```python
from build123d import *

# Parameters (mm, degrees)
SKETCH_1_W          = 40.5
SKETCH_1_H          = 20.25
EXTRUDE_1_DEPTH     = 9
CUT_EXTRUDE_START   = -1
SKETCH_2_R          = 9.25
CUT_EXTRUDE_1_DEPTH = 9
SKETCH_3_W          = 6.125
SKETCH_3_H          = 8
SKETCH_3_W_2        = 8
SKETCH_3_W_3        = 12.25
SKETCH_3_H_2        = 6.125
CUT_EXTRUDE_2_DEPTH = 1
CHAMFER_1_SIZE      = 1
SKETCH_4_R          = 1.1
SKETCH_4_R_2        = 0.7
SKETCH_4_R_3        = 0.9
SKETCH_4_R_4        = 0.5
CUT_EXTRUDE_3_DEPTH = 7.2
EXTRUDE_2_DEPTH     = 7.8
CUT_EXTRUDE_4_DEPTH = 7.8
FILLET_1_R          = 0.3


with BuildPart() as part:
    # Эскиз1 → Бобышка-Вытянуть1 (new body)
    with BuildSketch(Plane.XY):
        Rectangle(SKETCH_1_W, SKETCH_1_H)
    extrude(amount=EXTRUDE_1_DEPTH)

    # Эскиз2 → Вырез-Вытянуть1 (cut)
    with BuildSketch(Plane.XY.offset(9).offset(CUT_EXTRUDE_START)):
        with Locations((-10.125, 0)):
            Circle(SKETCH_2_R)
        with Locations((10.125, 0)):
            Circle(SKETCH_2_R)
    extrude(amount=-CUT_EXTRUDE_1_DEPTH, mode=Mode.SUBTRACT)

    # Эскиз3 → Вырез-Вытянуть2 (cut)
    with BuildSketch(Plane.XY.offset(9)):
        with Locations((-17.1875, 0)):
            Rectangle(SKETCH_3_W, SKETCH_3_H)
        with Locations((-10.125, 0)):
            Rectangle(SKETCH_3_W_2, SKETCH_3_H)
        Rectangle(SKETCH_3_W_3, SKETCH_3_H)
        with Locations((10.125, 0)):
            Rectangle(SKETCH_3_W_2, SKETCH_3_H)
        with Locations((17.1875, 0)):
            Rectangle(SKETCH_3_W, SKETCH_3_H)
        with Locations((10.125, 7.0625)):
            Rectangle(SKETCH_3_W_2, SKETCH_3_H_2)
        with Locations((-10.125, 7.0625)):
            Rectangle(SKETCH_3_W_2, SKETCH_3_H_2)
        with Locations((-10.125, -7.0625)):
            Rectangle(SKETCH_3_W_2, SKETCH_3_H_2)
        with Locations((10.125, -7.0625)):
            Rectangle(SKETCH_3_W_2, SKETCH_3_H_2)
    extrude(amount=-CUT_EXTRUDE_2_DEPTH, mode=Mode.SUBTRACT)

    # Фаска1
    chamfer_1_edges = [part.edges().sort_by_distance(p)[0] for p in [
        (-14.125, 4, 8.5),
        (-6.125, 4, 8.5),
        (6.125, 4, 8.5),
        (14.125, 4, 8.5),
        (14.125, -4, 8.5),
        (6.125, -4, 8.5),
        (-6.125, -4, 8.5),
        (-14.125, -4, 8.5),
    ]]
    chamfer(chamfer_1_edges, length=CHAMFER_1_SIZE)

    # Эскиз4 → Вырез-Вытянуть3 (cut)
    with BuildSketch(Plane.XY.offset(9)):
        with Locations((-18.55, 7.925)):
            Circle(SKETCH_4_R)
        with Locations((-18.95, -6.925)):
            Circle(SKETCH_4_R_2)
        with Locations((16.85, 8.625)):
            Circle(SKETCH_4_R_3)
        with Locations((17.45, -7.525)):
            Circle(SKETCH_4_R_4)
        with BuildLine():
            Line((3.079897776, 8.675), (0.433012702, 4.09046057))
            ThreePointArc((0.433012702, 4.09046057), (0, 3.84046057), (-0.433012702, 4.09046057))
            Line((-0.433012702, 4.09046057), (-3.079897776, 8.675))
            ThreePointArc((-3.079897776, 8.675), (-3.079897776, 9.175), (-2.646885074, 9.425))
            Line((-2.646885074, 9.425), (2.646885074, 9.425))
            ThreePointArc((2.646885074, 9.425), (3.079897776, 9.175), (3.079897776, 8.675))
        make_face()
        with BuildLine():
            Line((-0.346410162, -4.14), (-2.003589838, -7.010319398))
            ThreePointArc((-2.003589838, -7.010319398), (-2.003589838, -7.410319398), (-1.657179677, -7.610319398))
            Line((-1.657179677, -7.610319398), (1.657179677, -7.610319398))
            ThreePointArc((1.657179677, -7.610319398), (2.003589838, -7.410319398), (2.003589838, -7.010319398))
            Line((2.003589838, -7.010319398), (0.346410162, -4.14))
            ThreePointArc((0.346410162, -4.14), (0, -3.94), (-0.346410162, -4.14))
        make_face()
    extrude(amount=-CUT_EXTRUDE_3_DEPTH, mode=Mode.SUBTRACT)

    # Эскиз5 → Бобышка-Вытянуть2 (add)
    with BuildSketch(Plane(origin=(0, 0, 0), x_dir=(-1, 0, 0), z_dir=(0, 0, -1))):
        Polygon((-14.165851779, 11.625), (-17.165851779, 11.625), (-16.565851779, 10.125), (-14.765851779, 10.125), align=None)
        Polygon((-6.084148221, 11.625), (-5.484148221, 10.125), (-3.684148221, 10.125), (-3.084148221, 11.625), align=None)
        Polygon((6.084148221, 11.625), (3.084148221, 11.625), (3.684148221, 10.125), (5.484148221, 10.125), align=None)
        Polygon((14.165851779, 11.625), (14.765851779, 10.125), (16.565851779, 10.125), (17.165851779, 11.625), align=None)
        Polygon((20.25, 7.4), (20.25, 5.6), (21.75, 5), (21.75, 8), align=None)
        Polygon((20.25, -7.4), (21.75, -8), (21.75, -5), (20.25, -5.6), align=None)
    extrude(amount=-EXTRUDE_2_DEPTH)

    # Эскиз6 → Вырез-Вытянуть4 (cut)
    with BuildSketch(Plane(origin=(0, 0, 0), x_dir=(-1, 0, 0), z_dir=(0, 0, -1))):
        Polygon((17.365851779, -8.425), (16.665851779, -10.125), (14.665851779, -10.125), (13.965851779, -8.425), align=None)
        Polygon((6.284148221, -8.425), (2.884148221, -8.425), (3.584148221, -10.125), (5.584148221, -10.125), align=None)
        Polygon((-16.665851779, -10.125), (-14.665851779, -10.125), (-13.965851779, -8.425), (-17.365851779, -8.425), align=None)
        Polygon((-2.884148221, -8.425), (-3.584148221, -10.125), (-5.584148221, -10.125), (-6.284148221, -8.425), align=None)
        Polygon((-18.55, -4.739111724), (-18.55, -8.139111724), (-20.25, -7.439111724), (-20.25, -5.439111724), align=None)
        Polygon((-18.55, 8.139111724), (-20.25, 7.439111724), (-20.25, 5.439111724), (-18.55, 4.739111724), align=None)
    extrude(amount=-CUT_EXTRUDE_4_DEPTH, mode=Mode.SUBTRACT)

    # Скругление1
    fillet_1_edges = [part.edges().sort_by_distance(p)[0] for p in [
        (-20.25, 7.0625, 9),
        (-17.1875, -10.125, 9),
        (20.25, 7.0625, 9),
        (0, 10.125, 9),
        (-17.1875, 10.125, 9),
        (-20.25, -7.0625, 9),
        (0, -10.125, 9),
        (17.1875, -10.125, 9),
        (20.25, -7.0625, 9),
        (17.1875, 10.125, 9),
        (20.25, -10.125, 4.5),
        (-20.25, -10.125, 4.5),
        (-20.25, 10.125, 4.5),
        (20.25, 10.125, 4.5),
    ]]
    fillet(fillet_1_edges, radius=FILLET_1_R)


solid = part.part
```
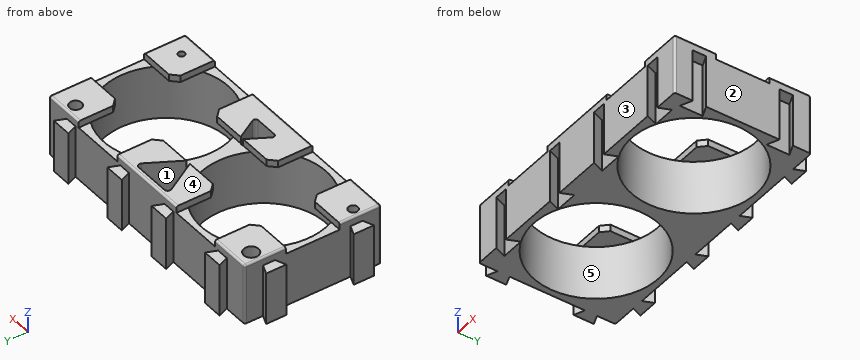
Read the model definition and answer for the solid it produces. Units are mm, in the model's axes. Face numbers are marked on the shaded views. A direction names the side the tool comes from. Coordinates: 2 decimals unless noted, no trailing zeros. Write each loop counter-clockwise with the first axis right and the second up, starting at its lowest first coordinate (ties: lowest second). Pieces come first, ordered by that corner, then holes. Notation, with made-up numbers: (9.25, 85) -> (53.25, 85) arc R23 cw to (53.25, 110) -> close; hole circle Ø11 at (43.25, 57.5). An arc over 180 degrees is marked (long way). Return JSON: item names as keys, results as strings.
1. A cutting plane is placed at C-C (x = -13.5). Determine the outline of the cut face in (y, z) (3 decimals).
Found:
{"outline": "(-10.125, 0) -> (-8.612, 0) -> (-8.612, 8) -> (-10.125, 8) -> close; (8.612, 0) -> (10.125, 0) -> (10.125, 8) -> (8.612, 8) -> close"}
2. A cutting plane is placed at B-B (x = -7). Determine the outline of the cut face in (y, z) (3 decimals), and give its area (3 significant figures).
Found:
{"outline": "(-10.125, 0) -> (-8.706, 0) -> (-8.706, 8) -> (-10.125, 8) -> close; (8.706, 0) -> (10.125, 0) -> (10.125, 8) -> (8.706, 8) -> close", "area": "22.7 mm2"}
3. A tool of negligible diameter and unlimited length cuts with its end or side. For the marked faces 4 and 5, from which of +Z, -Z, +X, -X, +Y, -Y can it reach the whole face along a straight path? Write none if from no direction.
Found:
{"face 4": "+Z, +X, -X, +Y, -Y", "face 5": "-Z"}
4. Find the intervals of material crossed by line 1 along X through (y, z) = (4, 5.75); line 2 along X through (y, z) = (1, 1.75); line 3 along Y through (x, z) = (-18.55, 6) (3 decimals), in increasing order. Write a range as from..to.
Found:
{"line 1": "-20.25..-18.47, -1.78..-0.37, 0.37..1.78, 18.47..20.25", "line 2": "-20.25..-19.32, -0.93..0.93, 19.32..20.25", "line 3": "-10.125..-7.499, -6.351..-3.819, 3.819..6.825, 9.025..10.125"}
5. Determine the mould class of the marked faces 1, 2 and 3 for opening direction Y: pulls with the +Y half, pulls with the -Y half, needs draft (parallel to the pull), parting line crosses it, or undercut.
Found:
{"face 1": "undercut", "face 2": "needs draft", "face 3": "pulls with the -Y half"}
6. Each of these flat-tipped pins is pushed along its axis until it touches: P1, Ø1.3, axis at x = -15.5, y = -6.5, coming from the -Z side; P2, Ø10, axis at x = -6, y = 4, coming from the -Z side; P3, Ø0.5, axis at x = -2, z = 8.5, coming from the +Y side (3 decimals); P4, Ø0.8, axis at y = -7.5, z = 8.5, coming from the -X side. Where does it stop, or does it pass through?
Found:
{"P1": "z = 8", "P2": "z = 0", "P3": "y = 10.125", "P4": "x = -20.25"}
7. A cutting plane is placed at A-A (y = 0). Determine the outline of the cut face in (x, z) (3 decimals), and give its area (3 significant figures).
Found:
{"outline": "(-20.25, 0) -> (-19.375, 0) -> (-19.375, 8) -> (-20.25, 8) -> close; (-0.875, 0) -> (0.875, 0) -> (0.875, 8) -> (-0.875, 8) -> close; (19.375, 0) -> (20.25, 0) -> (20.25, 8) -> (19.375, 8) -> close", "area": "28.0 mm2"}
8. A cutting plane is placed at D-D (z = 4.5). Give the number of separate pieces and of enclosed holes in the cut face, and give its area (3 significant figures).
Found:
{"separate pieces": "1", "enclosed holes": "8", "area": "238 mm2"}
